Can you work these out from the model? Positions are in its coordinate system, mm. Face numbers are marked on the shaded views. A direction names the side the tool comes from. Coordinates: 2 decimals unless noted, no trailing zeros. Order: outer loops, then holes, each group sorted by start corner. A loop starts at its lowest first (then second) coordinate and runs counter-clockwise, first axis right, second up. Notation, with made-up numbers: (11.5, 35.25) - (52.5, 35.25) arc R22 cw to (52.5, 72.25) - close; hole circle Ø5 at (-18.75, -2.5). An arc over 180 degrees is marked (long way). Use a Markdown table: item, result. Add a question column.
(1) We'd pull the mould along X, two halves only. Please class the marked faces 1, 2 and 3: pulls with the +X half, pulls with the -X half, needs draft (parallel to the pull), parting line crosses it, or undercut.
(2) On a 3-axis mill with a long thin cutter (end or side, diameter ignored), from which of +Z, -Z, +X, -X, +Y, -Y can I reach the whole of each face in a straight line? I mean the marked faces 4 and 5. Say none if no direction works.
(3) I want a section at B-B (y = 24). List the corners of the cut face in (x, z) for me.
(4) I want a section at D-D (x = 0). List the corners of the cut face in (y, z) for me, and give its area (3 significant figures).
(5) I want a section at A-A (z = 0). List the corners of the cut face in (x, y) for me, and give its area (3 significant figures).
(6) For pin 1 Ø12 at (x, y) = (-17, 14.5) entering from -Z; pin 2 Ø1 at (x, y) = (10, 9.5) entering from -Z; pin 3 Ø3 at (y, z) = (8.5, 15) entering from +X, each with a flat end and sliding along its axis, tell me the tip position at first contact or that it passes through.
(7) I want a section at C-C (z = 8.5). List the corners of the cut face in (x, y) for me, and give its area (3 significant figures).
(8) If I drill on L1, parallel to X at y = 11, z = 0; L2, parallel to X at y = 21.5, z = 12.5; L3, parallel to Y at x = 17, z = 1, over which ranges is the centre line in solid material (lowest first)? Write a range as [from, to].
```python
from build123d import *

# Parameters (mm, degrees)
SKETCH1_R               = 32.5
BOSS_EXTRUDE1_DEPTH     = 15
SKETCH2_R               = 17
BOSS_EXTRUDE2_DEPTH     = 13
CUT_EXTRUDE2_DEPTH      = 54.819141576
CUT_EXTRUDE2_DEPTH_BACK = 54.819141576
SKETCH3_R               = 1.55
CUT_EXTRUDE3_DEPTH      = 54.819141576


with BuildPart() as part:
    # Sketch1 → Boss-Extrude1 (new body)
    with BuildSketch(Plane(origin=(0, 0, 0), x_dir=(1, 0, 0), z_dir=(0, 1, 0))):
        with Locations(Location((0, 0, 0), (0, 0, 270))):
            Circle(SKETCH1_R)
    extrude(amount=BOSS_EXTRUDE1_DEPTH)

    # Sketch2 → Boss-Extrude2 (add)
    with BuildSketch(Plane(origin=(0, 15, 0), x_dir=(1, 0, 0), z_dir=(0, 1, 0))):
        with Locations(Location((0, 0, 0), (0, 0, 90))):
            Circle(SKETCH2_R)
    extrude(amount=BOSS_EXTRUDE2_DEPTH)

    # Sketch3 → Cut-Extrude2 (cut, two sides: drawn at the far end of the back side and taken through both)
    with BuildSketch(Plane.XY.offset(-CUT_EXTRUDE2_DEPTH_BACK)):
        with Locations((0.022370376, 21.5)):
            Circle(SKETCH3_R)
    extrude(amount=CUT_EXTRUDE2_DEPTH + CUT_EXTRUDE2_DEPTH_BACK, mode=Mode.SUBTRACT)

    # Sketch4 → Cut-Extrude3 (cut, through all)
    with BuildSketch(Plane(origin=(0, 28, 0), x_dir=(1, 0, 0), z_dir=(0, 1, 0))):
        with BuildLine():
            Line((-2.948304598, 4.1), (2.948304598, 4.1))
            ThreePointArc((2.948304598, 4.1), (0, -5.05), (-2.948304598, 4.1))
        make_face()
    extrude(amount=-CUT_EXTRUDE3_DEPTH, mode=Mode.SUBTRACT)


solid = part.part
```
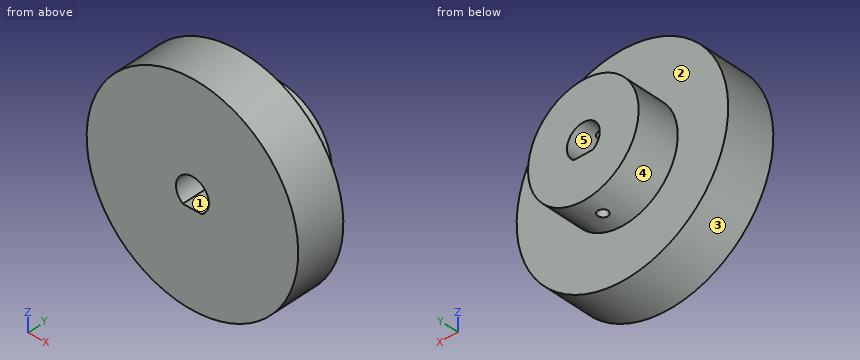
Answers follow:
| question | item | result |
|---|---|---|
| 1 | face 1 | undercut |
| 1 | face 2 | needs draft |
| 1 | face 3 | parting line crosses it |
| 2 | face 4 | +Y |
| 2 | face 5 | +Y, -Y |
| 3 | outline | circle Ø34 at (0, 0); hole (-2.95, -4.1) - (2.95, -4.1) arc R5.05 ccw (long way) to start |
| 4 | outline | (0, -32.5) - (15, -32.5) - (15, -17) - (19.95, -17) - (19.95, -4.1) - (0, -4.1) - close; (0, 5.05) - (19.95, 5.05) - (19.95, 17) - (15, 17) - (15, 32.5) - (0, 32.5) - close; (23.05, -17) - (28, -17) - (28, -4.1) - (23.05, -4.1) - close; (23.05, 5.05) - (28, 5.05) - (28, 17) - (23.05, 17) - close |
| 4 | area | 1,080 mm² |
| 5 | outline | (-32.5, 0) - (-5.05, 0) - (-5.05, 28) - (-17, 28) - (-17, 15) - (-32.5, 15) - close; (5.05, 0) - (32.5, 0) - (32.5, 15) - (17, 15) - (17, 28) - (5.05, 28) - close |
| 5 | area | 1,130 mm² |
| 6 | pin 1 | stops at z = -30.58 |
| 6 | pin 2 | stops at z = -31.08 |
| 6 | pin 3 | stops at x = 29.56 |
| 7 | outline | (-31.37, 0) - (31.37, 0) - (31.37, 15) - (14.72, 15) - (14.72, 28) - (-14.72, 28) - (-14.72, 15) - (-31.37, 15) - close; hole circle Ø3.1 at (0.02, 21.5) |
| 7 | area | 1,320 mm² |
| 8 | L1 | x = [-32.5, -5.05], [5.05, 32.5] |
| 8 | L2 | x = [-11.52, -1.53], [1.57, 11.52] |
| 8 | L3 | y = [0, 15] |
